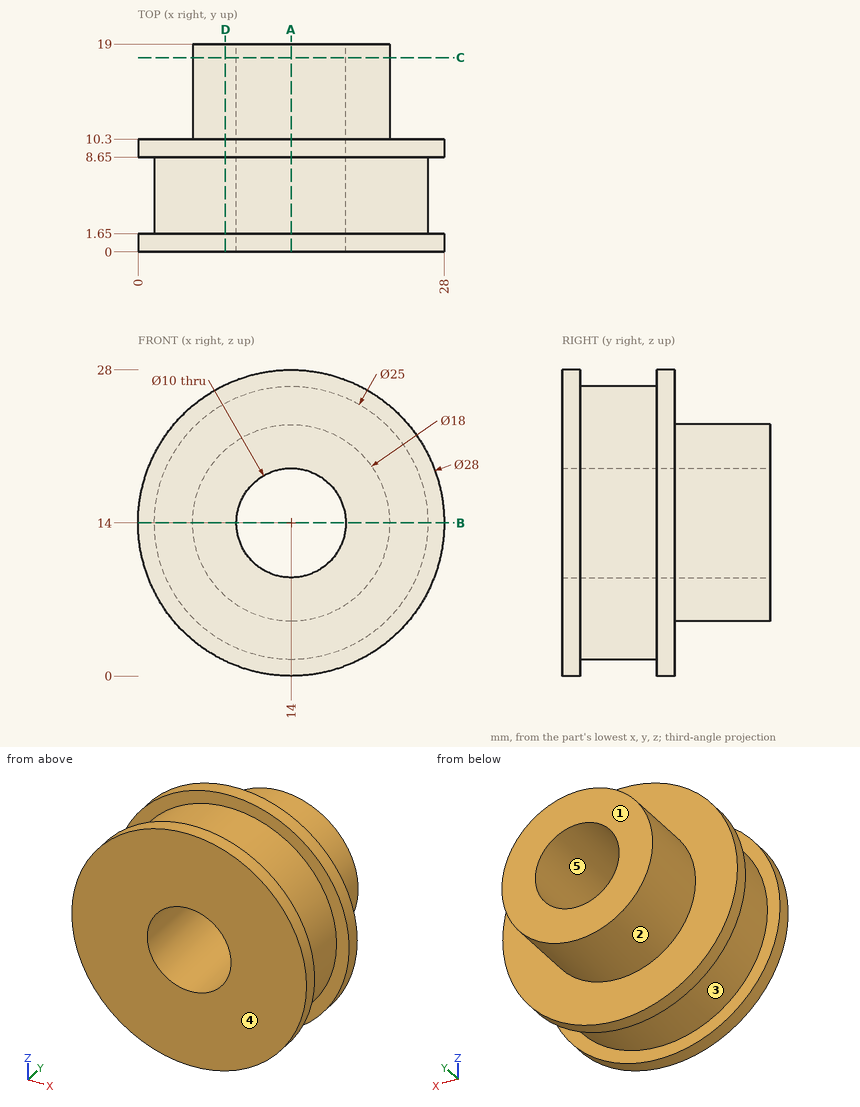
Check sheet for the drawn part. Datum: minimum x, y, z corner. Units: mm. A direction names the side the tool comes from. Round coordinates to 2 decimals unless told otherwise and drop trailing zeros. Write each loop counter-clockwise with the first axis right and the second up, starting at its lowest first coordinate (ties: lowest second). Pieces come first, ordered by that corner, then holes. Notation, with made-up numbers: (-26, -9.75) -> (22, -9.75) arc R16 cw to (22, 5.25) -> close; hole circle Ø7 at (32, -23). An arc over 180 degrees is marked (long way). One line per item, written item: value. Start each with the question number.
(1) Access from +Z, -Z, +X, -X, +Y, -Y to the whole of each face (thin tool, end or side, straight path). Record for the marked faces 1 and 2.
(2) Cross-section at B-B, the plane z = 14. Record the cut outline in (x, y).
(3) Cross-section at D-D, the plane x = 8. Record the cut outline in (y, z), and give its area (3 significant figures).
(4) Go/stop test with flat-tipped pins: pin 1 Ø1 at (x, y) = (16, 6) entering from -Z; pin 2 Ø10 at (y, z) = (12.5, 3) entering from +X; pin 3 Ø6 at (x, y) = (18, 2) entering from -Z. Record where each tip stops, or that it passes through.
(5) Draft check along Z on the marked faces 3, 4 and 5. Enter one of: +Z half, -Z half, draft (parallel to the pull), parting line (faces both ways), or undercut.
(6) Cross-section at C-C, the plane y = 17.75. Record the cut outline in (x, z), and give its area (3 significant figures).
(7) Scan lines: line 1 (X direction, y = 6, z = 14); line 2 (Z direction, x = 14, y = 13.5); line 3 (X direction, y = 9.75, z = 14). Record each from-to range of solid material in increasing order. Write a range as [from, to].
(8) Cross-section at A-A, the plane x = 14. Record the cut outline in (y, z).
Answer:
1. face 1: +Z, -Z, +X, -X, +Y
1. face 2: +Y
2. outline: (0, 0) -> (9, 0) -> (9, 19) -> (5, 19) -> (5, 10.3) -> (0, 10.3) -> (0, 8.65) -> (1.5, 8.65) -> (1.5, 1.65) -> (0, 1.65) -> close; (19, 0) -> (28, 0) -> (28, 1.65) -> (26.5, 1.65) -> (26.5, 8.65) -> (28, 8.65) -> (28, 10.3) -> (23, 10.3) -> (23, 19) -> (19, 19) -> close
3. outline: (0, 1.35) -> (1.65, 1.35) -> (1.65, 3.03) -> (8.65, 3.03) -> (8.65, 1.35) -> (10.3, 1.35) -> (10.3, 7.29) -> (19, 7.29) -> (19, 20.71) -> (10.3, 20.71) -> (10.3, 26.65) -> (8.65, 26.65) -> (8.65, 24.97) -> (1.65, 24.97) -> (1.65, 26.65) -> (0, 26.65) -> close
3. area: 354 mm²
4. pin 1: z = 1.59
4. pin 2: x = 26.39
4. pin 3: z = 0.04
5. face 3: parting line
5. face 4: draft
5. face 5: undercut
6. outline: circle Ø18 at (14, 14); hole circle Ø10 at (14, 14)
6. area: 176 mm²
7. line 1: [1.5, 9], [19, 26.5]
7. line 2: [5, 9], [19, 23]
7. line 3: [0, 9], [19, 28]
8. outline: (0, 0) -> (1.65, 0) -> (1.65, 1.5) -> (8.65, 1.5) -> (8.65, 0) -> (10.3, 0) -> (10.3, 5) -> (19, 5) -> (19, 9) -> (0, 9) -> close; (0, 19) -> (19, 19) -> (19, 23) -> (10.3, 23) -> (10.3, 28) -> (8.65, 28) -> (8.65, 26.5) -> (1.65, 26.5) -> (1.65, 28) -> (0, 28) -> close
